```python
from build123d import *

# Parameters (mm, degrees)
SKETCH2_R           = 20.15
BOSS_EXTRUDE1_DEPTH = 30


with BuildPart() as part:
    # Sketch2 → Boss-Extrude1 (new body)
    with BuildSketch(Plane(origin=(0, 0, 0), x_dir=(1, 0, 0), z_dir=(0, 1, 0))):
        with BuildLine():
            Line((36.829871123, -10), (36.829871123, 4))
            Line((36.829871123, 4), (24.829871123, 4))
            ThreePointArc((24.829871123, 4), (0, 25.15), (-24.829871123, 4))
            Line((-24.829871123, 4), (-36.829871123, 4))
            Line((-36.829871123, 4), (-36.829871123, -10))
            Line((-36.829871123, -10), (-23.076449034, -10))
            ThreePointArc((-23.076449034, -10), (-16.228725969, -19.213301471), (-6, -24.423810104))
            Line((-6, -24.423810104), (-6, -84.423810104))
            Line((-6, -84.423810104), (6, -84.423810104))
            Line((6, -84.423810104), (6, -24.423810104))
            ThreePointArc((6, -24.423810104), (16.228725969, -19.213301471), (23.076449034, -10))
            Line((23.076449034, -10), (36.829871123, -10))
        make_face()
        with Locations(Location((0, 0, 0), (0, 0, 270))):
            Circle(SKETCH2_R, mode=Mode.SUBTRACT)
    extrude(amount=BOSS_EXTRUDE1_DEPTH)


solid = part.part
```
The model under review builds one solid part; all positions refer to its coordinate system, in mm. A direction names the side the tool comes from. Round coordinates to 2 decimals unless told otherwise and drop trailing zeros. Order: outer loops, then holes, each group sorted by start corner. A loop starts at its lowest first (then second) coordinate and runs counter-clockwise, first axis right, second up. Notation, with made-up numbers: M 4.5,21 L 36.5,21 A29 cw 36.5,53 Z; hole C -23.5,3 d1. An arc over 180 degrees is marked long. Use a Markdown table: item, result.
1) Insertion check: pin 1 (4 mm diameter, centred on y = 13.5, z = 41.5, fed in from -X); pin 2 (12 mm diameter, centred on y = 12.5, z = -14, fed in from +X); pin 3 (10 mm diameter, centred on x = 26.5, y = 17.5, fed in from +Z). Each pin has a flat end and moves straight along its axis. Give the tip position at first contact, or say it passes through.
Report:
| item | result |
|---|---|
| pin 1 | x = -6 |
| pin 2 | x = 23.84 |
| pin 3 | z = 13.05 |
2) Draft analysis for pull direction X (two halves, no side actions). For faces 1 (the face through (6, 15, 55)), 2 (the face through (31, 15, -4)), 3 (the face through (-19.67, 14.79, -4.37)), state which applies: released by +X, released by -X, zero draft, split by the parting line, or undercut.
Report:
| item | result |
|---|---|
| face 1 | released by +X |
| face 2 | zero draft |
| face 3 | undercut |
3) Consider section B-B (y = 22). Write out the cut boundary in (x, z), then the cut area to 3 significant figures.
Report:
| item | result |
|---|---|
| outline | M -36.83,-4 L -24.83,-4 A25.15 ccw 24.83,-4 L 36.83,-4 L 36.83,10 L 23.08,10 A25.15 ccw 6,24.42 L 6,84.42 L -6,84.42 L -6,24.42 A25.15 ccw -23.08,10 L -36.83,10 Z; hole C 0,0 d40.3 |
| area | 1,770 mm^2 |
4) Wall thickness on line 1 along X through (y, z) = (13, 0); line 2 along X through (y, z) = (3.75, 29); line 3 along X through (y, z) = (5.5, -15.5): over which ranges is each line inside the solid? List them lowest first. Write a range as [from, to].
Report:
| item | result |
|---|---|
| line 1 | [-36.83, -20.15], [20.15, 36.83] |
| line 2 | [-6, 6] |
| line 3 | [-19.81, -12.88], [12.88, 19.81] |
5) Consider section C-C (z = 0). Write out the cut boundary in (x, y).
Report:
| item | result |
|---|---|
| outline | M -36.83,0 L -20.15,0 L -20.15,30 L -36.83,30 Z; M 20.15,0 L 36.83,0 L 36.83,30 L 20.15,30 Z |
6) Consider section D-D (z = 35.5). Write out the cut boundary in (x, y).
Report:
| item | result |
|---|---|
| outline | M -6,0 L 6,0 L 6,30 L -6,30 Z |
7) Consider section A-A (x = 0). Write out the cut boundary in (y, z), then the cut area to 3 significant figures.
Report:
| item | result |
|---|---|
| outline | M 0,-25.15 L 30,-25.15 L 30,-20.15 L 0,-20.15 Z; M 0,20.15 L 30,20.15 L 30,84.42 L 0,84.42 Z |
| area | 2,080 mm^2 |
8) Tool access review of faces 4 (the face through (30, 15, 10)), 5 (the face through (-31, 15, -4)), 6 (the face through (-30, 15, 10)): name each direction out of +Z, -Z, +X, -X, +Y, -Y from which nothing blocks a thin tool from reaching the whole face with its end or side.
Report:
| item | result |
|---|---|
| face 4 | +Z, +X, +Y, -Y |
| face 5 | -Z, -X, +Y, -Y |
| face 6 | +Z, -X, +Y, -Y |
